Part model, mm, in its own coordinate system. Face numbers are marked on the shaded views. A direction names the side the tool comes from. Round coordinates to 2 decimals unless told otherwise and drop trailing zeros. Loops run counter-clockwise (first coordinate to the right, second up) from the corner with the lowest first, then second, coordinate; pieces in that order, holes last.
1) Band-saw the part on C-C, the plane z = -19.5. Write the cut outline in (x, y), then the cut area to 3 significant figures.
2) Band-saw the part on A-A, the plane y = 0. Write the cut outline in (x, z), then the cut area to 3 significant figures.
3) Drop flat-ended pins along their axis: P1, Ø1.7, axis at x = -1, y = 38, coming from the +Z side; P2, Ø16.5, axis at x = -2, z = -16.5, coming from the +Y side; P3, Ø2, axis at x = -18.5, z = 1, coming from the +Y side; P4, Ø2, axis at x = -28.5, y = 10.5, coming from the -Z side. Give the stop position or say it passes through.
4) Probe line 1 (Y direction, x = 0, z = 1.5); line 2 (Y direction, x = 28.5, z = 6.25). List the from-to ranges inside material, lowest first.
5) Mould opens along X. For the marked faces 4, 5 and 6 say: +X half, -X half, draft (parallel to the pull), parting line (faces both ways), or undercut.
6) 3-axis set-ups, long thin cutter, end or side, ignore diameter. For the marked faces 1, 2 and 3: which of +Z, -Z, +X, -X, +Y, -Y reach the whole face in a straight line?
7) Band-saw the part on B-B, the plane z = -3.25. Write the cut outline in (x, y).
from build123d import *

# Parameters (mm, degrees)
BOSS_EXTRUDE1_DEPTH      = 7.5
SKETCH6_W                = 15
SKETCH6_H                = 4
BOSS_EXTRUDE2_DEPTH      = 15
FILLET1_R                = 7.5
CIRPATTERN1_COUNT        = 3
FILLET1_OF_CIRPATTERN1_R = 7.5


with BuildPart() as part:
    # Sketch2 → Revolve1 (revolve)
    with BuildSketch(Plane(origin=(0, 0, 0), x_dir=(1, 0, 0), z_dir=(0, 1, 0))):
        Polygon((37, 0), (37, -7.5), (32, -7.5), (32, 7.5), (39.009618943, 7.5), align=None)
    revolve(axis=Axis((0, 0, 7.5), (0, 0, -1)))

    # Sketch3 → Boss-Extrude1 (add)
    with BuildSketch(Plane(origin=(0, 0, -7.5), x_dir=(-1, 0, 0), z_dir=(0, 0, -1))):
        with BuildLine():
            Line((-2.5, 38.929428073), (-2.5, 33.929428073))
            Line((-2.5, 33.929428073), (2.5, 33.929428073))
            Line((2.5, 33.929428073), (2.5, 38.929428073))
            ThreePointArc((2.5, 38.929428073), (0, 39.009618943), (-2.5, 38.929428073))
        make_face()
    boss_extrude1 = extrude(amount=-BOSS_EXTRUDE1_DEPTH)

    # Sketch6 → Boss-Extrude2 (add)
    with BuildSketch(Plane(origin=(0, 0, -7.5), x_dir=(-1, 0, 0), z_dir=(0, 0, -1))):
        with Locations((0, 36.281854319)):
            Rectangle(SKETCH6_W, SKETCH6_H)
    boss_extrude2 = extrude(amount=BOSS_EXTRUDE2_DEPTH)

    # Fillet1
    fillet1_edges = [part.edges().sort_by_distance(p)[0] for p in [
        (-7.5, 36.281854319, -22.5),
        (7.5, 36.281854319, -22.5),
    ]]
    fillet(fillet1_edges, radius=FILLET1_R - 0.0001)  # a hair under: the kernel refuses the full size

    # CirPattern1: Boss-Extrude1, Boss-Extrude2 ×3 about axis
    cirpattern1_axis = Axis((0, 0, 0), (0, 0, 1))
    add([boss_extrude1.rotate(cirpattern1_axis, i * 360 / CIRPATTERN1_COUNT) for i in range(1, CIRPATTERN1_COUNT)])
    add([boss_extrude2.rotate(cirpattern1_axis, i * 360 / CIRPATTERN1_COUNT) for i in range(1, CIRPATTERN1_COUNT)])

    # Fillet1 of CirPattern1
    fillet1_of_cirpattern1_edges = [part.edges().sort_by_distance(p)[0] for p in [
        (-27.671007537, -24.636117688, -22.5),
        (-35.171007537, -11.645736631, -22.5),
        (35.171007537, -11.645736631, -22.5),
        (27.671007537, -24.636117688, -22.5),
    ]]
    fillet(fillet1_of_cirpattern1_edges, radius=FILLET1_OF_CIRPATTERN1_R - 0.0001)  # a hair under: the kernel refuses the full size


solid = part.part
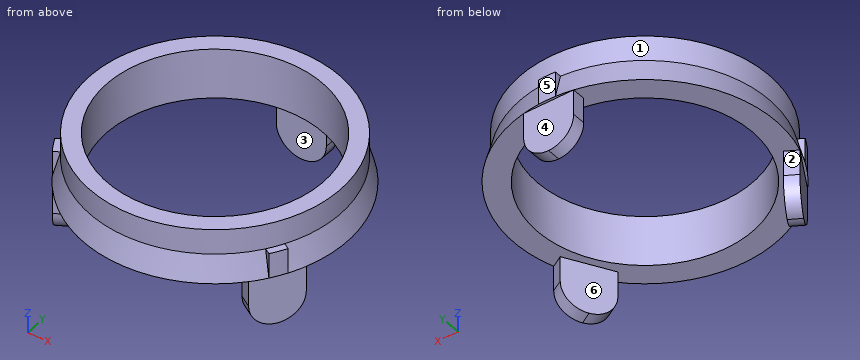
Reported:
1. outline: (-36.15, -13.94) - (-30.15, -24.34) - (-26.69, -22.34) - (-32.69, -11.94) - close; (-6, 34.28) - (6, 34.28) - (6, 38.28) - (-6, 38.28) - close; (26.69, -22.34) - (30.15, -24.34) - (36.15, -13.94) - (32.69, -11.94) - close
1. area: 144 mm2
2. outline: (-39.01, -7.5) - (-32, -7.5) - (-32, 7.5) - (-37, 7.5) - (-37, 0) - close; (32, -7.5) - (39.01, -7.5) - (37, 0) - (37, 7.5) - (32, 7.5) - close
2. area: 165 mm2
3. P1: stops at z = 0
3. P2: stops at y = 38.28
3. P3: stops at y = 32.6
3. P4: passes through
4. line 1: y = -37 to -32, 32 to 37
4. line 2: y = -23.6 to -14.55, 14.55 to 23.6
5. face 4: draft
5. face 5: parting line
5. face 6: undercut
6. face 1: +Z
6. face 2: -Z, -X, +Y
6. face 3: -Z, +X, -X, -Y
7. outline: (-34.96, -17.3) arc R39.01 ccw to (-32.46, -21.63) - (-31.48, -21.06) arc R37.87 ccw to (31.48, -21.06) - (32.46, -21.63) arc R39.01 ccw to (34.96, -17.3) - (33.98, -16.73) arc R37.87 ccw to (2.5, 37.79) - (2.5, 38.93) arc R39.01 ccw to (-2.5, 38.93) - (-2.5, 37.79) arc R37.87 ccw to (-33.98, -16.73) - close; hole circle Ø64 at (0, 0)
